from build123d import *

# Parameters (mm, degrees)
F0_R     = 24
F1_DEPTH = 240
F2_SIZE  = 1
F5_W     = 50
F5_H     = 41
F6_DEPTH = 125
F8_D     = 17.5


with BuildPart() as f1:
    # F0 (on Front) → F1 (new body)
    with BuildSketch(Plane.XZ):
        Circle(F0_R)
    extrude(amount=F1_DEPTH)

    # F2
    f2_edges = [f1.edges().sort_by_distance(p)[0] for p in [
        (24, -120, 0),
        (-24, 0, 0),
        (-24, -240, 0),
    ]]
    chamfer(f2_edges, length=F2_SIZE)

    # F5 (on offset) → F6 (cut)
    with BuildSketch(Plane.XY.offset(8)):
        with Locations((0, -20.5)):
            Rectangle(F5_W, F5_H)
        with Locations((0, -219.5)):
            Rectangle(F5_W, F5_H)
    extrude(amount=F6_DEPTH, mode=Mode.SUBTRACT)

    # F8 (through all)
    with Locations(Plane.XY.offset(8)):
        with Locations((0, -20.5), (0, -219.5)):
            Hole(F8_D / 2)


solid = f1.part
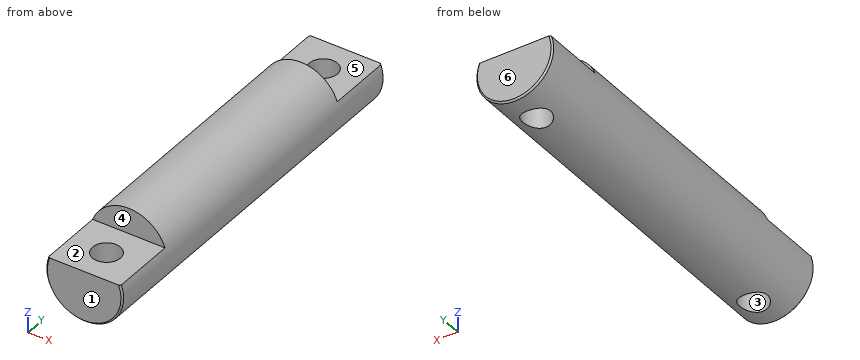
Can you work these out from the model? Positions are in its coordinate system, mm. Face numbers are marked on the shaded views. A direction names the side the tool comes from. Coordinates: 2 decimals unless noted, no trailing zeros. Order: outer loops, then holes, each group sorted by start corner. A loop starts at its lowest first (then second) coordinate and runs counter-clockwise, first axis right, second up. Notation, with made-up numbers: (73, 73) - (114, 73) arc R9 cw to (114, 77) - close; hole circle Ø7 at (-7.75, -31.75). An arc over 180 degrees is marked (long way). Answer as a JSON object with one key per item and string values. Group by question number.
Q1. Imagine slicing it at D-D (y = -100.5). Please give me the cut outline in (x, z), and give its area (3 significant figures).
Q2. I need wall thicknesses on line 1 (Y direction, x = 0, z = -6); line 2 (X direction, y = -20.5, z = 1); line 3 (Y direction, x = 15.5, z = 12.5). Which ranges of each line are inside material? Lowest first, please. Write a range as from..to.
Q3. Imagine slicing it at C-C (y = -20.5). Please give me the cut outline in (x, z), and give its area (3 significant figures).
Q4. On a 3-axis mill with a long thin cutter (end or side, diameter ignored), from which of +Z, -Z, +X, -X, +Y, -Y can I reach the whole of each face in a straight line? I mean the marked faces 4, 5 and 6. Say none if no direction works.
Q5. Imagine slicing it at A-A (z = 0). Please give me the cut outline in (x, y).
Q6. We'd pull the mould along Y, two halves only. Please class the marked faces 1, 2 and 3: +Y half, -Y half, draft (parallel to the pull), parting line (faces both ways), or undercut.
Q7. Will these pins go through, and if not, where does the flat tip stop? P1, Ø20.5, axis at x = 7.5, y = -14.5, coming from the +Z side; P2, Ø10.5, axis at x = 0, y = -219.5, coming from the -Z side; P3, Ø6, axis at x = -1, z = -16.5, coming from the +Y side; P4, Ø2, axis at x = 1, y = -133.5, coming from the +Z side.
Q8. Imagine slicing it at B-B (x = 0). Please give me the cut outline in (y, z).
Determined:
{
 "1": {"outline": "circle Ø48 at (0, 0)", "area": "1,810 mm2"},
 "2": {"line 1": "y = -240..-228.25, -210.75..-29.25, -11.75..0", "line 2": "x = -23.98..-8.75, 8.75..23.98", "line 3": "y = -199..-41"},
 "3": {"outline": "(-22.63, 8) arc R24 ccw to (-8.75, -22.35) - (-8.75, 8) - close; (8.75, -22.35) arc R24 ccw to (22.63, 8) - (8.75, 8) - close", "area": "731 mm2"},
 "4": {"face 4": "+Z, +X, -X, -Y", "face 5": "+Z, +X, -X, +Y", "face 6": "+Z, -Z, +X, -X, +Y"},
 "5": {"outline": "(-24, -239) - (-23, -240) - (23, -240) - (24, -239) - (24, -1) - (23, 0) - (-23, 0) - (-24, -1) - close; hole circle Ø17.5 at (0, -219.5); hole circle Ø17.5 at (0, -20.5)"},
 "6": {"face 1": "-Y half", "face 2": "draft", "face 3": "undercut"},
 "7": {"P1": "stops at z = 8", "P2": "passes through", "P3": "stops at y = 0", "P4": "stops at z = 24"},
 "8": {"outline": "(-240, -23) - (-239, -24) - (-228.25, -24) - (-228.25, 8) - (-240, 8) - close; (-210.75, -24) - (-29.25, -24) - (-29.25, 8) - (-41, 8) - (-41, 24) - (-199, 24) - (-199, 8) - (-210.75, 8) - close; (-11.75, -24) - (-1, -24) - (0, -23) - (0, 8) - (-11.75, 8) - close"}
}
